```python
from build123d import *

# Parameters (mm, degrees)
BOSS_EXTRUDE1_DEPTH = 3
SKETCH2_R           = 1.9
SKETCH2_R_2         = 6.25
CUT_EXTRUDE1_DEPTH  = 4
BOSS_EXTRUDE3_DEPTH = 143.5
SKETCH6_W           = 47
SKETCH6_H           = 16
CUT_EXTRUDE4_DEPTH  = 3
SKETCH7_R           = 1.9
CUT_EXTRUDE5_DEPTH  = 94


with BuildPart() as part:
    # Sketch1 → Boss-Extrude1 (new body)
    with BuildSketch(Plane.XY):
        with BuildLine():
            Line((0, 0), (143.5, 0))
            Line((143.5, 0), (143.5, -25))
            ThreePointArc((143.5, -25), (145.839555569, -31.427876097), (151.763518223, -34.84807753))
            Line((151.763518223, -34.84807753), (191.155828344, -41.794004637))
            ThreePointArc((191.155828344, -41.794004637), (199.235618402, -49.733992213), (194.718539209, -60.122563128))
            Line((194.718539209, -60.122563128), (149.336384129, -88.480480962))
            ThreePointArc((149.336384129, -88.480480962), (146.793565045, -89.612616959), (144.037191487, -90))
            Line((144.037191487, -90), (-35.962808513, -90))
            ThreePointArc((-35.962808513, -90), (-43.033876325, -87.071067812), (-45.962808513, -80))
            Line((-45.962808513, -80), (-45.962808513, -70))
            ThreePointArc((-45.962808513, -70), (-44.396722971, -64.627003917), (-40.18899113, -60.93692213))
            Line((-40.18899113, -60.93692213), (-1.99069399, -43.124763645))
            ThreePointArc((-1.99069399, -43.124763645), (-0.539954223, -41.852499015), (0, -40))
            Line((0, -40), (0, 0))
        make_face()
    extrude(amount=BOSS_EXTRUDE1_DEPTH)

    # Sketch2 → Cut-Extrude1 (cut, through all)
    with BuildSketch(Plane.XY.offset(3)):
        with Locations((185.228339525, -47.568848131)):
            Circle(SKETCH2_R)
        with Locations((132.107823371, -80.5)):
            Circle(SKETCH2_R)
        with Locations((76.307823371, -80.5)):
            Circle(SKETCH2_R)
        with Locations((21.107823371, -80.5)):
            Circle(SKETCH2_R)
        with Locations((102.5, -27.75)):
            Circle(SKETCH2_R_2)
        with Locations((131.007823371, -17.5)):
            Circle(SKETCH2_R)
        with BuildLine():
            Line((-32.167176629, -82.4), (-37.617176629, -82.4))
            ThreePointArc((-37.617176629, -82.4), (-39.517176629, -80.5), (-37.617176629, -78.6))
            Line((-37.617176629, -78.6), (-32.167176629, -78.6))
            ThreePointArc((-32.167176629, -78.6), (-30.267176629, -80.5), (-32.167176629, -82.4))
        make_face()
    extrude(amount=-CUT_EXTRUDE1_DEPTH, mode=Mode.SUBTRACT)

    # Sketch3 → Boss-Extrude3 (add)
    with BuildSketch(Plane(origin=(143.5, 0, 0), x_dir=(0, 0, -1), z_dir=(1, 0, 0))):
        with BuildLine():
            Line((-3, 0), (0, 0))
            ThreePointArc((0, 0), (-0.878679656, 2.121320344), (-3, 3))
            Line((-3, 3), (-16, 3))
            Line((-16, 3), (-16, 0))
            Line((-16, 0), (-3, 0))
        make_face()
    extrude(amount=-BOSS_EXTRUDE3_DEPTH)

    # Sketch6 → Cut-Extrude4 (cut)
    with BuildSketch(Plane(origin=(0, 3, 0), x_dir=(1, 0, 0), z_dir=(0, 1, 0))):
        with Locations((71, -8)):
            Rectangle(SKETCH6_W, SKETCH6_H)
    extrude(amount=-CUT_EXTRUDE4_DEPTH, mode=Mode.SUBTRACT)

    # Sketch7 → Cut-Extrude5 (cut, through all)
    with BuildSketch(Plane(origin=(0, 3, 0), x_dir=(1, 0, 0), z_dir=(0, 1, 0))):
        with Locations((133.6, -13)):
            Circle(SKETCH7_R)
        with Locations((104.4, -13)):
            Circle(SKETCH7_R)
        with Locations((37.6, -13)):
            Circle(SKETCH7_R)
        with Locations((8.4, -13)):
            Circle(SKETCH7_R)
    extrude(amount=-CUT_EXTRUDE5_DEPTH, mode=Mode.SUBTRACT)


solid = part.part
```
The listing builds one solid part. Answer for the finished solid, in the listing's coordinates (mm). A direction names the side the tool comes from. Coordinates: 2 decimals unless noted, no trailing zeros. Write each loop counter-clockwise with the first axis right and the second up, starting at its lowest first coordinate (ties: lowest second). Pieces come first, ordered by that corner, then holes. Notation, with made-up numbers: (17, 41.25) - (75, 41.25) arc R31 ccw to (75, 70.25) - close; hole circle Ø11 at (-37.5, 48). An arc over 180 degrees is marked (long way). One line per item, written item: value.
1) A tool of negligible diameter and unlimited length cuts with its end or side. For faces 1 (the flat face through (143.5, -5.7, 2.7)), 2 (the flat face through (0, -12, 2.7)), 3 (the flat face through (24, 3, 9)), 4 (the flat face through (78, -54, 3)), from which of +Z, -Z, +X, -X, +Y, -Y can it reach the whole face along a straight path? Write none if from no direction.
Geometry check:
face 1: +Z, -Z, +X, +Y
face 2: +Z, -Z, -X, +Y
face 3: +Z, -Z, +X, -X, +Y
face 4: +Z, +X, -X, -Y
2) Find section B-B (y = -12.5). Give the vertices of the cut face in (x, z).
Geometry check:
outline: (0, 0) - (143.5, 0) - (143.5, 3) - (0, 3) - close
3) Find section C-C (x = 81). Give the vertices of the cut face in (y, z), and give its area (3 significant figures).
Geometry check:
outline: (-90, 0) - (0, 0) - (0, 3) - (-90, 3) - close
area: 270 mm2
4) For a pull along X with two mould halves and no side action, classify faces 5 (the flat face through (78, -54, 0)), 6 (the flat face through (171.18, -38.27, 1.48)), 7 (the cylindrical face through (108.46, -25.87, 1.52)) as pulls with the +X half, pulls with the -X half, needs draft (parallel to the pull), parting line crosses it, or undercut.
Geometry check:
face 5: needs draft
face 6: pulls with the +X half
face 7: undercut
5) Find section A-A (z = 8.75). Give the vertices of the cut face in (x, y), and give its area (4 significant figures).
Geometry check:
outline: (0, 0) - (47.5, 0) - (47.5, 3) - (0, 3) - close; (94.5, 0) - (143.5, 0) - (143.5, 3) - (94.5, 3) - close
area: 289.5 mm2
6) Each of these flat-tipped pins is pushed along its axis until it touches: pin 1 Ø5 at (x, y) = (76.31, -80.5) entering from -Z; pin 2 Ø6 at (x, y) = (21.11, -80.5) entering from +Z; pin 3 Ø1.5 at (x, z) = (-35, 1) entering from +Y; pin 4 Ø3.5 at (x, z) = (71.5, 1.5) entering from +Y. Where does it stop, or does it pass through?
Geometry check:
pin 1: stops at z = 0
pin 2: stops at z = 3
pin 3: stops at y = -58.17
pin 4: stops at y = 0
7) Consider line 1 along X through (y, z) = (1.25, 13); line 2 along Z through (x, y) = (54, -66). Determine where each line is inside the solid, lowest interval first. Write a range as from..to.
Geometry check:
line 1: x = 0..6.5, 10.3..35.7, 39.5..47.5, 94.5..102.5, 106.3..131.7, 135.5..143.5
line 2: z = 0..3
